Read the model definition and answer for the solid it produces. Units are mm, in the model's axes. A direction names the side the tool comes from. Give positions to 0.01 mm unless a question says otherwise; leave off trailing zeros. Write each loop counter-clockwise with the first axis right and the second up, starting at its lowest first coordinate (ties: lowest second). Pieces come first, ordered by that corner, then holes. Notation, with made-up numbers: M 6.25,11.25 L 26.25,11.25 A16 cw 26.25,19.25 Z; hole C -3.75,39 d3. An arc over 180 degrees is marked long. Use a Markdown table: item, result. Add a question column.
Item 1: A cutting plane is placed at A-A on y = 7.5. Determine the outline of the cut face in (x, z) (3 decimals).
Item 2: For faces 1 (the flat face through (151, 5, 8)), 2 (the flat face through (152, 10, 4)), determine the directions among +Z, -Z, +X, -X, +Y, -Y from which every point of the face is accessible in a straight line to the end or side of a thin tool.
Item 3: Given P1, Ø6, axis at x = 149.225, z = 6.7, coming from the +Y side, flat-ended and moving along its own axis, determine where the tip first touches the part or whether it passes through.
Item 4: A cutting plane is placed at D-D on y = 3.25. Determine the outline of the cut face in (x, z) (3 decimals), then the cut area to 3 significant figures.
Item 5: Consider probe 1 along X at (y, z) = (7.1, 6.7) (3 decimals); probe 2 along X at (y, z) = (2.05, 6.7) (3 decimals); probe 3 along Y at (x, z) = (150.5, 4). Determine where each line is inside the solid, lowest interval first. Write a range as [from, to].
Item 6: The mould has two halves that part along Z. Classify faces 3 (the cylindrical face through (152.16, 7.46, 4.45)), 4 (the flat face through (160, 5, 7)), 5 (the flat face through (150, 5, 13.4)): pulls with the +Z half, pulls with the -Z half, needs draft (parallel to the pull), parting line crosses it, or undercut.
Item 7: A cutting plane is placed at C-C on x = 150. Determine the outline of the cut face in (y, z), then the cut area to 3 significant figures.
Item 8: A cutting plane is placed at B-B on z = 7.25. Determine the outline of the cut face in (x, y).
from build123d import *

# Parameters (mm, degrees)
PAD_DEPTH              = 13.4
CYLINDER_W             = 6.7
CYLINDER_H             = 298.45
CYLINDER_ANGLE         = 180
CYLINDER001_R          = 99.483333
CYLINDER001_DEPTH      = 32
BOX_W                  = 149.225
BOX_H                  = 30
BOX_DEPTH              = 21
BOX001_W               = 33
BOX001_H               = 149.225
BOX001_DEPTH           = 22
CYLINDER002_R          = 3.7
CYLINDER002_DEPTH      = 105
LINEARPATTERN_COUNT    = 3
LINEARPATTERN_PITCH    = 74.6125
CYLINDER003_R          = 1.85
CYLINDER003_DEPTH      = 100
LINEARPATTERN001_COUNT = 3
LINEARPATTERN001_PITCH = 74.6125
CYLINDER004_R          = 2.55
CYLINDER004_DEPTH      = 10
LINEARPATTERN002_COUNT = 3
LINEARPATTERN002_PITCH = 141.16875
BOX002_W               = 100
BOX002_H               = 1000
BOX002_DEPTH           = 100
BOX003_W               = 100
BOX003_H               = 100
BOX003_DEPTH           = 1000
BOX004_W               = 50
BOX004_H               = 100
BOX004_DEPTH           = 100
BOX005_W               = 500
BOX005_H               = 500
BOX005_DEPTH           = 500
BOX006_W               = 37
BOX006_H               = 26
BOX006_DEPTH           = 16


with BuildPart() as part:
    # Sketch → Pad (new body)
    with BuildSketch(Plane.XY):
        Polygon((0, 0), (298.45, 0), (0, 298.45), align=None)
    extrude(amount=PAD_DEPTH)

    # Cylinder → Cylinder (revolve, cut)
    with BuildSketch(Plane(origin=(0, 0, 6.7), x_dir=(0, 0, 1), z_dir=(-1, 0, 0))):
        with Locations((3.35, 149.225)):
            Rectangle(CYLINDER_W, CYLINDER_H)
    revolve(axis=Axis((0, 0, 6.7), (0, 1, 0)), revolution_arc=CYLINDER_ANGLE, mode=Mode.SUBTRACT)

    # Cylinder001 → Cylinder001 (cut)
    with BuildSketch(Plane(origin=(149.225, 149.225, -8), x_dir=(1, 0, 0), z_dir=(0, 0, 1))):
        Circle(CYLINDER001_R)
    extrude(amount=CYLINDER001_DEPTH, mode=Mode.SUBTRACT)

    # Box → Box (cut)
    with BuildSketch(Plane(origin=(149.225, 79.741667, 17), x_dir=(1, 0, 0), z_dir=(0, 0, -1))):
        with Locations((74.6125, 15)):
            Rectangle(BOX_W, BOX_H)
    extrude(amount=BOX_DEPTH, mode=Mode.SUBTRACT)

    # Box001 → Box001 (cut)
    with BuildSketch(Plane(origin=(49.741667, 303.579167, 17), x_dir=(1, 0, 0), z_dir=(0, 0, -1))):
        with Locations((16.5, 74.6125)):
            Rectangle(BOX001_W, BOX001_H)
    extrude(amount=BOX001_DEPTH, mode=Mode.SUBTRACT)

    # Cylinder002 → Cylinder002 (cut)
    with BuildSketch(Plane(origin=(74.6125, 5, 6.7), x_dir=(-1, 0, 0), z_dir=(0, 1, 0))):
        Circle(CYLINDER002_R)
    cylinder002 = extrude(amount=CYLINDER002_DEPTH, mode=Mode.SUBTRACT)

    # LinearPattern: Cylinder002 ×3
    with Locations(*[(i * LINEARPATTERN_PITCH, 0, 0) for i in range(1, LINEARPATTERN_COUNT)]):
        add(cylinder002, mode=Mode.SUBTRACT)

    # Cylinder003 → Cylinder003 (cut)
    with BuildSketch(Plane(origin=(74.6125, 0, 6.7), x_dir=(-1, 0, 0), z_dir=(0, 1, 0))):
        Circle(CYLINDER003_R)
    cylinder003 = extrude(amount=CYLINDER003_DEPTH, mode=Mode.SUBTRACT)

    # LinearPattern001: Cylinder003 ×3
    with Locations(*[(i * LINEARPATTERN001_PITCH, 0, 0) for i in range(1, LINEARPATTERN001_COUNT)]):
        add(cylinder003, mode=Mode.SUBTRACT)

    # Cylinder004 → Cylinder004 (cut)
    with BuildSketch(Plane(origin=(0, 8.05625, 5), x_dir=(1, 0, 0), z_dir=(0, 0, 1))):
        Circle(CYLINDER004_R)
    cylinder004 = extrude(amount=CYLINDER004_DEPTH, mode=Mode.SUBTRACT)

    # LinearPattern002: Cylinder004 ×3
    with Locations(*[(0, i * LINEARPATTERN002_PITCH, 0) for i in range(1, LINEARPATTERN002_COUNT)]):
        add(cylinder004, mode=Mode.SUBTRACT)

    # Box002 → Box002 (cut)
    with BuildSketch(Plane.XY):
        with Locations((50, 500)):
            Rectangle(BOX002_W, BOX002_H)
    extrude(amount=BOX002_DEPTH, mode=Mode.SUBTRACT)

    # Box003 → Box003 (cut)
    with BuildSketch(Plane.YZ.offset(160)):
        with Locations((50, 50)):
            Rectangle(BOX003_W, BOX003_H)
    extrude(amount=BOX003_DEPTH, mode=Mode.SUBTRACT)

    # Box004 → Box004 (cut)
    with BuildSketch(Plane(origin=(90, 78, -74), x_dir=(1, 0, 0), z_dir=(0, -1, 0))):
        with Locations((25, 50)):
            Rectangle(BOX004_W, BOX004_H)
    extrude(amount=BOX004_DEPTH, mode=Mode.SUBTRACT)

    # Box005 → Box005 (cut)
    with BuildSketch(Plane(origin=(0, 25, 0), x_dir=(0, 1, 0), z_dir=(1, 0, 0))):
        with Locations((250, 250)):
            Rectangle(BOX005_W, BOX005_H)
    extrude(amount=BOX005_DEPTH, mode=Mode.SUBTRACT)

    # Box006 → Box006 (cut)
    with BuildSketch(Plane(origin=(136, 26, -5), x_dir=(1, 0, 0), z_dir=(0, -1, 0))):
        with Locations((18.5, 13)):
            Rectangle(BOX006_W, BOX006_H)
    extrude(amount=BOX006_DEPTH, mode=Mode.SUBTRACT)


solid = part.part
Filled in:
| question | item | result |
|---|---|---|
| 1 | outline | M 140,0 L 160,0 L 160,13.4 L 140,13.4 Z; hole C 149.225,6.7 d7.4 |
| 2 | face 1 | +Y |
| 2 | face 2 | +Z, -Z, +X, -X, +Y |
| 3 | P1 | y = 5 |
| 4 | outline | M 140,0 L 160,0 L 160,13.4 L 140,13.4 Z; hole C 149.225,6.7 d3.7 |
| 4 | area | 257 mm² |
| 5 | probe 1 | [140, 145.525], [152.925, 160] |
| 5 | probe 2 | [140, 147.375], [151.075, 160] |
| 5 | probe 3 | [0, 5] |
| 6 | face 3 | undercut |
| 6 | face 4 | needs draft |
| 6 | face 5 | pulls with the +Z half |
| 7 | outline | M 0,0 L 10,0 L 10,3.08 L 5,3.08 L 5,5.02 L 0,5.02 Z; M 0,8.38 L 5,8.38 L 5,10.32 L 10,10.32 L 10,13.4 L 0,13.4 Z |
| 7 | area | 81.0 mm² |
| 8 | outline | M 140,0 L 147.46,0 L 147.46,5 L 145.57,5 L 145.57,10 L 140,10 Z; M 150.99,0 L 160,0 L 160,10 L 152.88,10 L 152.88,5 L 150.99,5 Z |
